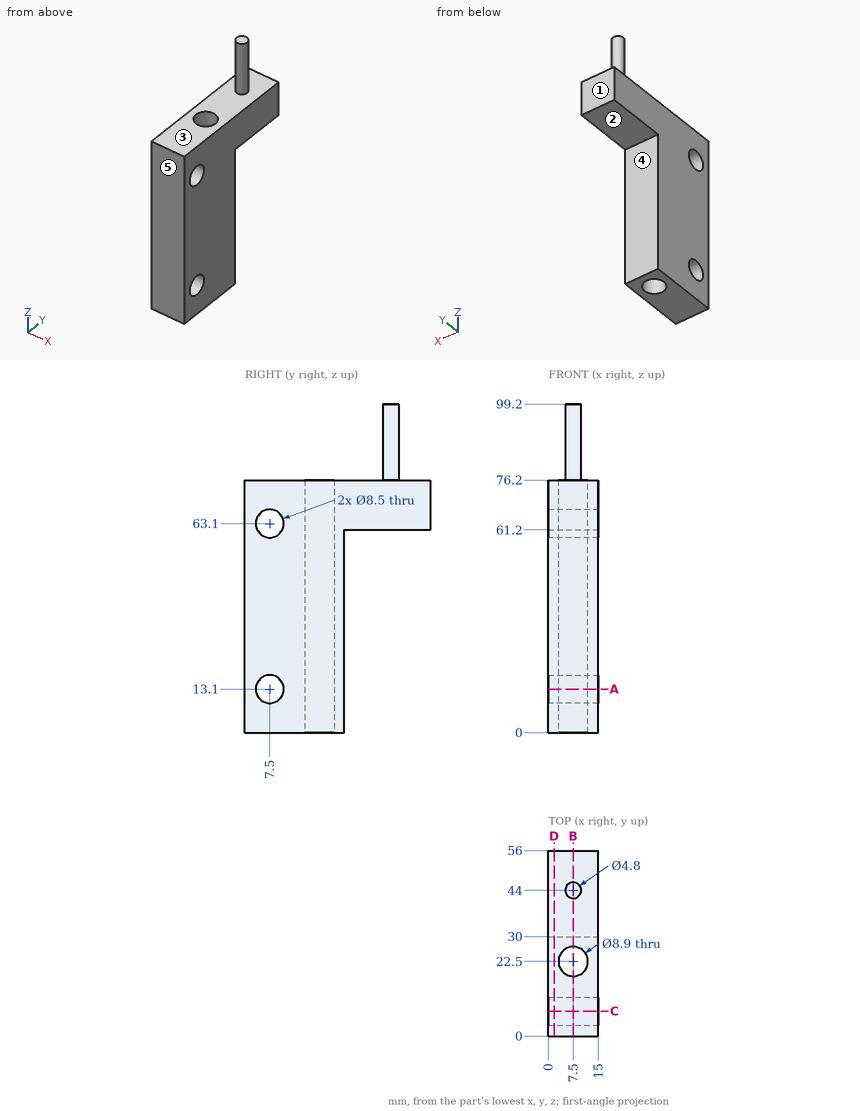
Geometry check sheet. Reference: drawing and pictorial views, mm from the part's lowest x, y, z. A direction names the side the tool comes from. Give positions to 0.01 mm unless a question says otherwise; leave off trailing zeros. Order: outer loops, then holes, each group sorted by start corner. A loop starts at its lowest first (then second) coordinate and runs counter-clockwise, first axis right, second up. Notation, with made-up numbers: M -19,-27.75 L 29,-27.75 A19 cw 29,-0.75 Z; hole C -39,57.25 d6. An arc over 180 degrees is marked long. Answer as CSV lines item,"result". Start each with the question number.
Item 1: Cross-section at D-D on x = 1.75. Enter the section's corners in (y, z).
Item 2: Gauge pin test, flat ends, axial feed: P1, Ø7, axis at y = 7.5, z = 63.1, coming from the -X side; P2, Ø6, axis at x = 9.5, y = 33.5, coming from the +Z side; P3, Ø4.5, axis at x = 11, y = 41, coming from the -Z side; P4, Ø1.5, axis at x = 3.5, z = 23.5, coming from the +Y side. Record the tip position at first contact, or that the pin passes through.
Item 3: Tool access check on the marked faces 4 and 5. Record the directions out of +Z, -Z, +X, -X, +Y, -Y that give a thin tool (end or side, any length) a straight path to the whole face; none if there is none.
Item 4: Mould release check, pull along Z, two halves, no side actions. Record for the marked faces 1, 2 and 3: +Z half, -Z half, draft (parallel to the pull), parting line (faces both ways), or undercut.
Item 5: Cross-section at A-A on z = 13.1. Enter the section's corners in (x, y).
Item 6: Thickness scan on line 1 (Y direction, x = 7, z = 12); line 2 (Y direction, x = 4.25, z = 63.1); line 3 (Y direction, x = 7.5, z = 20). Record the ranges inside material, lowest first. Write a range as [from, to].
Item 7: Cross-section at C-C on y = 7.5. Enter the section's corners in (x, z), plus the area to 3 significant figures.
Item 8: Cross-section at B-B on x = 7.5. Enter the section's corners in (y, z).
Established:
1,outline,"M 0,0 L 30,0 L 30,61.2 L 56,61.2 L 56,76.2 L 0,76.2 Z; hole C 7.5,13.1 d8.5; hole C 7.5,63.1 d8.5"
2,P1,"passes through"
2,P2,"stops at z = 76.2"
2,P3,"stops at z = 61.2"
2,P4,"stops at y = 30"
3,face 4,"-Z, +X, -X, +Y"
3,face 5,"+Z, -Z, +X, -X, -Y"
4,face 1,"draft"
4,face 2,"-Z half"
4,face 3,"+Z half"
5,outline,"M 0,0 L 15,0 L 15,3.25 L 0,3.25 Z; M 0,11.75 L 15,11.75 L 15,30 L 0,30 Z; hole C 7.5,22.5 d8.9"
6,line 1,"y = [0, 3.39], [11.61, 18.08], [26.92, 30]"
6,line 2,"y = [0, 3.25], [11.75, 19.46], [25.54, 56]"
6,line 3,"y = [0, 18.05], [26.95, 30]"
7,outline,"M 0,0 L 15,0 L 15,8.85 L 0,8.85 Z; M 0,17.35 L 15,17.35 L 15,58.85 L 0,58.85 Z; M 0,67.35 L 15,67.35 L 15,76.2 L 0,76.2 Z"
7,area,"888 mm^2"
8,outline,"M 0,0 L 18.05,0 L 18.05,76.2 L 0,76.2 Z; M 26.95,0 L 30,0 L 30,61.2 L 56,61.2 L 56,76.2 L 46.4,76.2 L 46.4,99.2 L 41.6,99.2 L 41.6,76.2 L 26.95,76.2 Z; hole C 7.5,13.1 d8.5; hole C 7.5,63.1 d8.5"
